Autodesk Inventor part; units mm, degrees
ref_plane "YZ Plane" through (0, 0, 0) normal (1, 0, 0) x (0, 1, 0)
ref_plane "XZ Plane" through (0, 0, 0) normal (0, 1, 0) x (-1, 0, 0)
ref_plane "XY Plane" through (0, 0, 0) normal (0, 0, 1) x (1, 0, 0)
sketch "スケッチ1" plane through (0, 0, 0) normal (0, 0, 1) x (1, 0, 0)
  circle A0 centre (0, 0) radius 30
  dimension "d0" = 60
extrude "押し出し1" add sketch "スケッチ1" along normal blind 40
sketch "スケッチ2" plane through (0, 0, 40) normal (0, 0, 1) x (1, 0, 0)
  circle A0 centre (0, 0) radius 27.5
  dimension "d3" = 55
extrude "押し出し2" cut sketch "スケッチ2" against normal blind 50
sketch "スケッチ3" plane through (0, 0, 0) normal (0, 0, 1) x (1, 0, 0)
  point P0 (0, 0)
sketch "スケッチ4" plane through (0, 0, 0) normal (1, 0, 0) x (0, 1, 0)
  line L0 (30, 0) -> (-30, 0)
  line L1 (-30, 0) -> (-30, 40)
  arc A0 (30, 0) -> (-30, 0) centre (0, 0) ccw
  dimension "d6" = 30
extrude "押し出し3" cut sketch "スケッチ4" along normal mid plane 50
sketch "スケッチ5" plane through (0, 0, 40) normal (0, 0, 1) x (1, 0, 0)
  circle A0 centre (0, 0) radius 27.5
extrude "押し出し4" add sketch "スケッチ5" against normal blind 1
sketch "スケッチ19" plane through (0, 0, 40) normal (0, 0, 1) x (1, 0, 0)
  circle A0 centre (0, 0) radius 27.5
  line L0 (27.5, -6.6575) -> (-27.5, -6.6575)
  line L1 (-27.5, -6.6575) -> (-27.5, 6.6575)
  line L2 (-27.5, 6.6575) -> (27.5, 6.6575)
  line L3 (27.5, 6.6575) -> (27.5, -6.6575)
  line L4 (27.5, -6.6575) -> (-27.5, 6.6575) construction
  line L5 (-27.5, -6.6575) -> (27.5, 6.6575) construction
  point P0 (26.682, -6.6575)
  point P1 (-26.682, -6.6575)
  point P2 (-26.682, 6.6575)
  point P3 (26.682, 6.6575)
extrude "押し出し11" cut sketch "スケッチ19" against normal blind 10 contours L2 A0 | A0 L0
sketch "スケッチ22" plane through (0, 0, 40) normal (0, 0, 1) x (1, 0, 0)
  point P0 (0, 0)
sketch "スケッチ23" plane through (0, 0, 40) normal (0, 0, 1) x (1, 0, 0)
  point P0 (0, 0)
  point P1 (-20, 0)
  point P2 (20, 0)
  dimension "d67" = 20
  dimension "d68" = 20
hole "穴4" at (-20, 0, 40) at (20, 0, 40) direction (0, 0, -1) diameter 3.2 depth 8.8 tip angle 118
sketch "スケッチ25" plane through (0, 0, 40) normal (0, 0, 1) x (1, 0, 0)
  point P0 (0, 0)
  point P1 (0, 0)
hole "穴5" at (0, 0, 40) direction (0, 0, -1) diameter 1.5 depth 8.8 tip angle 118
sketch "スケッチ26" plane through (0, 0, 40) normal (0, 0, 1) x (1, 0, 0)
  point P0 (0, 0)
  point P1 (-8.3, 0)
  point P2 (8.3, 0)
  dimension "d86" = 8.3
  dimension "d87" = 8.3
hole "穴6" at (-8.3, 0, 40) at (8.3, 0, 40) direction (0, 0, -1) diameter 3.2 depth 8.8 tip angle 118
properties part number "20220527_仮筒"
The listing builds one solid part. Answer for the finished solid, in the listing's coordinates (mm). A direction names the side the tool comes from. Give positions to 0.01 mm unless a question says otherwise; leave off trailing zeros. Write each loop counter-clockwise with the first axis right and the second up, starting at its lowest first coordinate (ties: lowest second). Pieces come first, ordered by that corner, then holes.
Item 1: Section D-D, the plane x = -20 is taken. Write down the section's boundary in (y, z).
Item 2: Which of the six approach directions +Z, -Z, +X, -X, +Y, -Y give full straight-line access (tool end or side, diameter ignored) to faces 1 (the cylindrical face through (-0.03, 0.75, 39.49)), 2 (the flat face through (0, 2, 39))?
Item 3: Determine the mould class of faces 3 (the flat face through (-28, 0, 0)), 4 (the cylindrical face through (28.615, -9.011, 24.164)), 5 (the cylindrical face through (26.23, 8.26, 24.72)) for opening direction Y: released by +Y, released by -Y, zero draft, split by the parting line, or undercut.
Item 4: Section C-C, the plane y = -22 is taken. Write down the section's boundary in (x, z).
Item 5: Find the intervals of material crossed by line 1 along Y through (x, z) = (0, 39.5); line 2 along Y through (x, z) = (8.3, 39.7); line 3 along Y through (x, z) = (0, 13), in increasing order.
Item 6: Flat-ended cylindrical pins translate along their axes: P1, Ø1, axis at x = 10.5, z = 14.5, coming from the -Y side; P2, Ø8, axis at y = -4, z = 14, coming from the -X side; P3, Ø1.5, axis at y = -14, z = 12, coming from the +X side; P4, Ø12, axis at x = -2, z = 31.5, coming from the -Y side. Find the tip coordinate at first contact, or state that the pin passes through.
Item 7: Section A-A, the plane z = 8 is taken. Write down the section's boundary in (x, y).
Item 8: Section B-B, the plane x = 23 is taken. Write down the section's boundary in (y, z).
Completed:
1. outline: (-22.36, 20) arc R30 cw to (-18.87, 23.32) - (-18.87, 40) - (-22.36, 40) - close; (-6.66, 39) - (-1.6, 39) - (-1.6, 40) - (-6.66, 40) - close; (1.6, 39) - (6.66, 39) - (6.66, 40) - (1.6, 40) - close; (18.87, 23.32) arc R30 cw to (22.36, 20) - (22.36, 40) - (18.87, 40) - close
2. face 1: +Z, -Z
2. face 2: -Z
3. face 3: zero draft
3. face 4: split by the parting line
3. face 5: undercut
4. outline: (-20.4, 20.4) - (-16.5, 20.4) - (-16.5, 40) - (-20.4, 40) - close; (16.5, 20.4) - (20.4, 20.4) - (20.4, 40) - (16.5, 40) - close
5. line 1: y = -30 to -27.5, -6.66 to -0.75, 0.75 to 6.66, 27.5 to 30
5. line 2: y = -28.83 to -26.22, -6.66 to -1.6, 1.6 to 6.66, 26.22 to 28.83
5. line 3: y = -30 to -27.5, 27.5 to 30
6. P1: stops at y = -28.28
6. P2: stops at x = -30
6. P3: stops at x = 26.92
6. P4: stops at y = -30
7. outline: (-25, -16.58) - (-25, -11.46) arc R27.5 cw to (-25, 11.46) - (-25, 16.58) arc R30 ccw to start; (-8, -28.91) arc R30 ccw to (8, -28.91) - close; (-8, 28.91) - (8, 28.91) arc R30 ccw to start; (25, -16.58) arc R30 ccw to (25, 16.58) - (25, 11.46) arc R27.5 cw to (25, -11.46) - close
8. outline: (-19.26, 23) arc R30 cw to (-15.07, 25.94) - (-15.07, 40) - (-19.26, 40) - close; (-6.66, 39) - (6.66, 39) - (6.66, 40) - (-6.66, 40) - close; (15.07, 25.94) arc R30 cw to (19.26, 23) - (19.26, 40) - (15.07, 40) - close
